Work out the finished part from the listing and answer in its coordinate system (mm). A direction names the side the tool comes from. Coordinates: 2 decimals unless noted, no trailing zeros. Order: outer loops, then holes, each group sorted by start corner. A loop starts at its lowest first (then second) coordinate and runs counter-clockwise, first axis right, second up. Notation, with made-up numbers: (12, -37) - (47, -37) arc R10 cw to (47, -24) - close; hole circle Ø6 at (1, -16.5). An arc over 180 degrees is marked (long way). Use CSV: the item, a comma, the result in double quotes. Start each with the question number.
from build123d import *

# Parameters (mm, degrees)
SKETCH1_R           = 9
SKETCH1_R_2         = 6
SKETCH1_R_3         = 4
BOSS_EXTRUDE1_DEPTH = 8
SKETCH3_R           = 8
SKETCH3_R_2         = 4
BOSS_EXTRUDE2_DEPTH = 3
SKETCH5_R           = 12
SKETCH5_R_2         = 6
BOSS_EXTRUDE3_DEPTH = 3
FILLET1_R           = 42


with BuildPart() as part:
    # Sketch1 → Boss-Extrude1 (new body)
    with BuildSketch(Plane(origin=(0, 0, 0), x_dir=(1, 0, 0), z_dir=(0, 1, 0))):
        with BuildLine():
            Line((82, 32.334641746), (14.735908192, 32.334641746))
            Line((14.735908192, 32.334641746), (-45.003147253, 56.470786852))
            ThreePointArc((-45.003147253, 56.470786852), (-54.304086029, 53.978607818), (-54.472135955, 44.351033997))
            Line((-54.472135955, 44.351033997), (-14.562305899, -10.580134541))
            ThreePointArc((-14.562305899, -10.580134541), (-5.562305899, -17.119017293), (5.562305899, -17.119017293))
            Line((5.562305899, -17.119017293), (85.708203932, 8.92196355))
            ThreePointArc((85.708203932, 8.92196355), (93.852260087, 22.211855326), (82, 32.334641746))
        make_face()
        Circle(SKETCH1_R, mode=Mode.SUBTRACT)
        with Locations((82, 20.334641746)):
            Circle(SKETCH1_R_2, mode=Mode.SUBTRACT)
        with Locations((-48, 49.053316016)):
            Circle(SKETCH1_R_3, mode=Mode.SUBTRACT)
    extrude(amount=BOSS_EXTRUDE1_DEPTH)

    # Sketch3 → Boss-Extrude2 (add, symmetric)
    with BuildSketch(Plane(origin=(-21.748054335, 0, -29.933628792), x_dir=(0.809016994, 0, -0.587785252), z_dir=(0.587785252, 0, 0.809016994))):
        with BuildLine():
            Line((-18, 46), (-18, 8))
            Line((-18, 8), (9.218720146, 8))
            Line((9.218720146, 8), (-2.309906432, 48.205098847))
            ThreePointArc((-2.309906432, 48.205098847), (-2.07785545, 47.113384808), (-2, 46))
            ThreePointArc((-2, 46), (-10, 38), (-18, 46))
        make_face()
        with Locations((-10, 46)):
            Circle(SKETCH3_R)
        with Locations((-10, 46)):
            Circle(SKETCH3_R_2, mode=Mode.SUBTRACT)
    extrude(amount=BOSS_EXTRUDE2_DEPTH, both=True)

    # Sketch5 → Boss-Extrude3 (add, symmetric)
    with BuildSketch(Plane(origin=(35.189091103, 0, -11.433628792), x_dir=(-0.309016994, 0, -0.951056516), z_dir=(0.951056516, 0, -0.309016994))):
        with BuildLine():
            Line((-18, 48), (-18, 8))
            Line((-18, 8), (14.770349605, 8))
            Line((14.770349605, 8), (5.737771209, 50.49494029))
            ThreePointArc((5.737771209, 50.49494029), (5.934262744, 49.254341559), (6, 48))
            ThreePointArc((6, 48), (-6, 36), (-18, 48))
        make_face()
        with Locations((-6, 48)):
            Circle(SKETCH5_R)
        with Locations((-6, 48)):
            Circle(SKETCH5_R_2, mode=Mode.SUBTRACT)
    extrude(amount=BOSS_EXTRUDE3_DEPTH, both=True)

    # Fillet1
    fillet1_edges = [part.edges().sort_by_distance(p)[0] for p in [
        (14.735908192, 4, -32.334641746),
    ]]
    fillet(fillet1_edges, radius=FILLET1_R)


solid = part.part
1) The part is cut by section C-C on y = 31. Determine the outline of the cut face in (x, z).
2) The part is cut by section A-A on y = 52. Determine the outline of the cut face in (x, z).
3) The part is cut by section B-B on x = -48. Determine the outline of the cut face in (y, z), plus the area to 3 significant figures.
4) The part is cut by section D-D on y = 6. Determine the outline of the cut face in (x, z).
5) Straight lines are drawn through the part: line 1 (Z direction, x = 82, y = 4.75); line 2 (Y direction, x = 26, z = -19); line 3 (Z direction, x = -48, y = 5.5). For each, find the intervals that lie inside material, in ascending order. Write a range as [from, to].
6) For faces 1 (the face through (-18.863, 27.821, -31.978)), 2 (the face through (53, 4, -32.335)), determine the directions among +Z, -Z, +X, -X, +Y, -Y from which every point of the face is accessible in a straight line to the end or side of a thin tool.
7) Flat-ended cylindrical pins translate along their axes: P1, Ø2, axis at y = 14.5, z = -8.5, coming from the +X side; P2, Ø23.5, axis at x = 0, z = 0, coming from the +Y side; P3, Ø8, axis at y = 15, z = 6, coming from the +X side; P4, Ø5, axis at x = -48, z = -49.05, coming from the -Y side. Find the tip coordinate at first contact, or state that the pin passes through.
8) For a pull along X with two mould halves and no side action, classify faces 3 (the face through (39.74, 28.59, -7.14)), 4 (the face through (-26.138, 26.211, -23.036)), 5 (the face through (32.04, 28.95, -21.26)), 6 (the face through (-29.664, 26.211, -27.89)) as +X half, -X half, draft (parallel to the pull), parting line (faces both ways), or undercut.
Answer key:
1,outline,"(-38.07, -21.78) - (-21.39, -33.9) - (-17.86, -29.05) - (-34.55, -16.93) - close; (29.28, -19.9) - (34.99, -21.76) - (43.6, 4.76) - (37.9, 6.61) - close"
2,outline,"(-35.88, -23.37) - (-27.32, -29.59) - (-23.79, -24.74) - (-32.36, -18.52) - close; (30.69, -15.56) - (36.4, -17.41) - (38.51, -10.91) - (32.81, -9.05) - close; (35.57, -0.55) - (41.28, -2.4) - (43.39, 4.11) - (37.69, 5.96) - close"
3,outline,"(0, -57.05) - (8, -57.05) - (8, -53.05) - (0, -53.05) - close; (0, -45.05) - (8, -45.05) - (8, -35.44) - (0, -35.44) - close"
3,area,"109 mm^2"
4,outline,"(-54.47, -44.35) arc R8 ccw to (-45, -56.47) - (7.17, -35.39) arc R42 cw to (22.9, -32.33) - (82, -32.33) arc R12 ccw to (85.71, -8.92) - (5.56, 17.12) arc R18 ccw to (-14.56, 10.58) - close; hole circle Ø8 at (-48, -49.05); hole circle Ø18 at (0, 0); hole circle Ø12 at (82, -20.33)"
5,line 1,"[-32.33, -26.33], [-14.33, -7.72]"
5,line 2,"[0, 8]"
5,line 3,"[-57.05, -53.05], [-45.05, -35.44]"
6,face 1,"-Z, +X, +Y"
6,face 2,"-Z, +X, +Y, -Y"
7,P1,"x = 39.62"
7,P2,"y = 8"
7,P3,"x = 43.6"
7,P4,"through"
8,face 3,"+X half"
8,face 4,"undercut"
8,face 5,"undercut"
8,face 6,"-X half"
